Input: dimensioned drawing with shaded views. Units: mm. Origin: part minimum x, y, z. Give positions to 0.01 mm unless a question says otherwise; leave off trailing zeros. Loops run counter-clockwise (first coordinate to the right, second up) from the corner with the lowest first, then second, coordinate; pieces in that order, holes last. Notation, with made-up numbers: (-20, -34.75) -> (-13, -34.75) arc R25 cw to (-13, -7.75) -> close; hole circle Ø7 at (32.5, 82.5). An arc over 180 degrees is marked (long way). Answer as a JSON object with one key per item and string values.
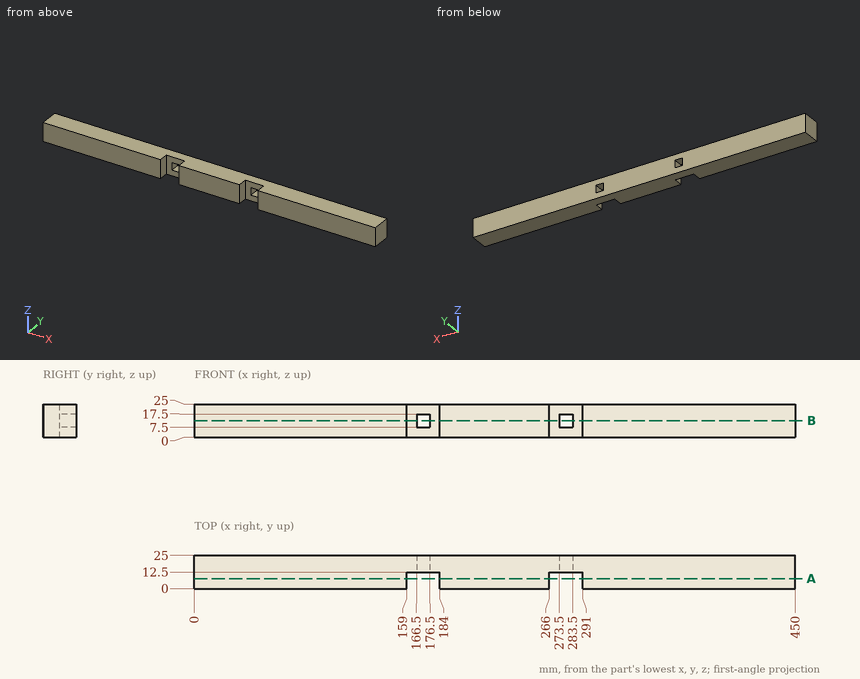
Q1. Ray query, line 1 along X through (y, z) = (12.25, 18); line 2 along X through (y, z) = (13, 16.25); line 3 along Z through (x, y) = (168.5, 17.75). Return the intervals inside material, ascending.
Evaluation:
{"line 1": "x = 0 to 159, 184 to 266, 291 to 450", "line 2": "x = 0 to 166.5, 176.5 to 273.5, 283.5 to 450", "line 3": "z = 0 to 7.5, 17.5 to 25"}
Q2. Pin query (flat end, axial travel): pin 1 (3 mm diameter, centred on x = 240, z = 19, fed in from -Y); pin 2 (7.5 mm diameter, centred on x = 279.5, z = 11.5, fed in from -Y). Return the tip coordinate at first contact, or that it passes through.
Evaluation:
{"pin 1": "stops at y = 0", "pin 2": "passes through"}
Q3. Section B-B, the plane z = 12.5. Return the cut outline in (x, y).
Evaluation:
{"outline": "(0, 0) -> (159, 0) -> (159, 12.5) -> (166.5, 12.5) -> (166.5, 25) -> (0, 25) -> close; (176.5, 12.5) -> (184, 12.5) -> (184, 0) -> (266, 0) -> (266, 12.5) -> (273.5, 12.5) -> (273.5, 25) -> (176.5, 25) -> close; (283.5, 12.5) -> (291, 12.5) -> (291, 0) -> (450, 0) -> (450, 25) -> (283.5, 25) -> close"}
Q4. Section A-A, the plane y = 7.5. Return the cut outline in (x, z), then the cut area to 3 significant figures.
Evaluation:
{"outline": "(0, 0) -> (159, 0) -> (159, 25) -> (0, 25) -> close; (184, 0) -> (266, 0) -> (266, 25) -> (184, 25) -> close; (291, 0) -> (450, 0) -> (450, 25) -> (291, 25) -> close", "area": "10,000 mm2"}
